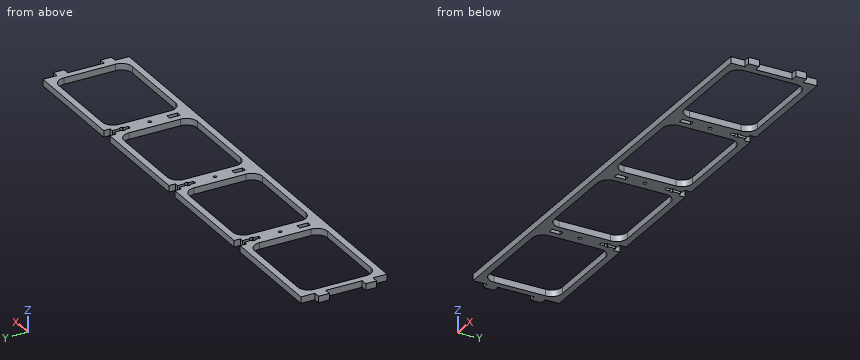
```python
from build123d import *

# Parameters (mm, degrees)
SKETCH1_W           = 428
SKETCH1_H           = 80
BOSS_EXTRUDE1_DEPTH = 6
CUT_EXTRUDE1_DEPTH  = 6
LPATTERN1_COUNT     = 4
LPATTERN1_PITCH     = 108.125
SKETCH3_R           = 1.6
SKETCH3_W           = 4.5
SKETCH3_H           = 10
CUT_EXTRUDE2_DEPTH  = 7
SKETCH4_W           = 6
SKETCH4_H           = 10
BOSS_EXTRUDE2_DEPTH = 6
SKETCH5_W           = 10
SKETCH5_H           = 6
CUT_EXTRUDE3_DEPTH  = 6
CUT_EXTRUDE4_REACH  = 8


with BuildPart() as part:
    # Sketch1 → Boss-Extrude1 (new body)
    with BuildSketch(Plane.XY):
        Rectangle(SKETCH1_W, SKETCH1_H)
    extrude(amount=BOSS_EXTRUDE1_DEPTH)

    # Sketch2 → Cut-Extrude1 (cut)
    with BuildSketch(Plane.XY.offset(6)):
        with BuildLine():
            Line((-116.375, -24), (-116.375, 24))
            ThreePointArc((-116.375, 24), (-119.303932188, 31.071067812), (-126.375, 34))
            Line((-126.375, 34), (-198, 34))
            ThreePointArc((-198, 34), (-205.071067812, 31.071067812), (-208, 24))
            Line((-208, 24), (-208, -24))
            ThreePointArc((-208, -24), (-205.071067812, -31.071067812), (-198, -34))
            Line((-198, -34), (-126.375, -34))
            ThreePointArc((-126.375, -34), (-119.303932188, -31.071067812), (-116.375, -24))
        make_face()
    cut_extrude1 = extrude(amount=-CUT_EXTRUDE1_DEPTH, mode=Mode.SUBTRACT)

    # LPattern1: Cut-Extrude1 ×4
    with Locations(*[(i * LPATTERN1_PITCH, 0, 0) for i in range(1, LPATTERN1_COUNT)]):
        add(cut_extrude1, mode=Mode.SUBTRACT)

    # Sketch3 → Cut-Extrude2 (cut, through all)
    with BuildSketch(Plane(origin=(0, 0, 0), x_dir=(-1, 0, 0), z_dir=(0, 0, -1))):
        with Locations((108.125, 0)):
            Circle(SKETCH3_R)
        Circle(SKETCH3_R)
        with Locations((-108.125, 0)):
            Circle(SKETCH3_R)
        with Locations((-108.125, -22)):
            Rectangle(SKETCH3_W, SKETCH3_H)
        with Locations((0, -22)):
            Rectangle(SKETCH3_W, SKETCH3_H)
        with Locations((108.125, -22)):
            Rectangle(SKETCH3_W, SKETCH3_H)
    extrude(amount=-CUT_EXTRUDE2_DEPTH, mode=Mode.SUBTRACT)

    # Sketch4 → Boss-Extrude2 (add)
    with BuildSketch(Plane(origin=(0, 0, 0), x_dir=(-1, 0, 0), z_dir=(0, 0, -1))):
        with Locations((-217, 22)):
            Rectangle(SKETCH4_W, SKETCH4_H)
        with Locations((-217, -22)):
            Rectangle(SKETCH4_W, SKETCH4_H)
        with Locations((217, -22)):
            Rectangle(SKETCH4_W, SKETCH4_H)
        with Locations((217, 22)):
            Rectangle(SKETCH4_W, SKETCH4_H)
    extrude(amount=-BOSS_EXTRUDE2_DEPTH)

    # Sketch5 → Cut-Extrude3 (cut)
    with BuildSketch(Plane(origin=(0, 40, 0), x_dir=(1, 0, 0), z_dir=(0, 1, 0))):
        with Locations((-108.125, -3)):
            Rectangle(SKETCH5_W, SKETCH5_H)
        with Locations((0, -3)):
            Rectangle(SKETCH5_W, SKETCH5_H)
        with Locations((108.125, -3)):
            Rectangle(SKETCH5_W, SKETCH5_H)
    extrude(amount=-CUT_EXTRUDE3_DEPTH, mode=Mode.SUBTRACT)

    # Sketch6 → Cut-Extrude4 (cut, up to next)
    with BuildSketch(Plane(origin=(0, 0, 0), x_dir=(-1, 0, 0), z_dir=(0, 0, -1)), mode=Mode.PRIVATE) as cut_extrude4_sk1:
        Polygon((-109.725, 34), (-109.725, 27), (-110.925, 27), (-110.925, 24), (-109.725, 24), (-109.725, 19), (-106.525, 19), (-106.525, 24), (-105.325, 24), (-105.325, 27), (-106.525, 27), (-106.525, 34), align=None)
    cut_extrude4_tool1 = extrude(cut_extrude4_sk1.sketch, amount=-CUT_EXTRUDE4_REACH, mode=Mode.PRIVATE) & part.part
    add(cut_extrude4_tool1.solids().sort_by_distance((108.125, 26.369565, 0))[0], mode=Mode.SUBTRACT)
    # Sketch6 → Cut-Extrude4 (cut, up to next)
    with BuildSketch(Plane(origin=(0, 0, 0), x_dir=(-1, 0, 0), z_dir=(0, 0, -1)), mode=Mode.PRIVATE) as cut_extrude4_sk2:
        Polygon((-1.595, 27), (-2.795, 27), (-2.795, 24), (-1.595, 24), (-1.595, 19), (1.605, 19), (1.605, 24), (2.805, 24), (2.805, 27), (1.605, 27), (1.605, 34), (-1.595, 34), align=None)
    cut_extrude4_tool2 = extrude(cut_extrude4_sk2.sketch, amount=-CUT_EXTRUDE4_REACH, mode=Mode.PRIVATE) & part.part
    add(cut_extrude4_tool2.solids().sort_by_distance((-0.005, 26.369565, 0))[0], mode=Mode.SUBTRACT)
    # Sketch6 → Cut-Extrude4 (cut, up to next)
    with BuildSketch(Plane(origin=(0, 0, 0), x_dir=(-1, 0, 0), z_dir=(0, 0, -1)), mode=Mode.PRIVATE) as cut_extrude4_sk3:
        Polygon((106.535, 34), (106.535, 27), (105.335, 27), (105.335, 24), (106.535, 24), (106.535, 19), (109.735, 19), (109.735, 24), (110.935, 24), (110.935, 27), (109.735, 27), (109.735, 34), align=None)
    cut_extrude4_tool3 = extrude(cut_extrude4_sk3.sketch, amount=-CUT_EXTRUDE4_REACH, mode=Mode.PRIVATE) & part.part
    add(cut_extrude4_tool3.solids().sort_by_distance((-108.135, 26.369565, 0))[0], mode=Mode.SUBTRACT)


solid = part.part
```
Geometry check sheet. Reference: the model listing, model coordinates, mm. Give positions to 0.01 mm unless a question says otherwise; leave off trailing zeros. Loops run counter-clockwise (first coordinate to the right, second up) from the corner with the lowest first, then second, coordinate; pieces in that order, holes last. Notation, with made-up numbers: M 36,4.25 L 66,4.25 A27 ccw 66,22.25 Z; hole C 28,86.25 d3. An arc over 180 degrees is marked long. Answer as CSV lines item,"result".
Item 1: Cross-section at B-B on z = 5.05. Count the separate pieces of the cut face and the enclosed holes in it, and give its area (3 significant figures).
Values:
separate pieces,"1"
enclosed holes,"10"
area,"9,400 mm²"
Item 2: Material ranges on line 1 (Y direction, x = 0, z = 1.8); line 2 (X direction, y = 14.5, z = 5) (3 decimals); line 3 (Y direction, x = -167, z = 0.85), recorded low to high.
Values:
line 1,"y = -40 to -27, -17 to -1.6, 1.6 to 19"
line 2,"x = -214 to -208, -116.375 to -99.875, -8.25 to 8.25, 99.875 to 116.375, 208 to 214"
line 3,"y = -40 to -34, 34 to 40"
Item 3: Cross-section at A-A on x = 178.5. Record the cut outline in (y, z).
Values:
outline,"M -40,0 L -34,0 L -34,6 L -40,6 Z; M 34,0 L 40,0 L 40,6 L 34,6 Z"
Item 4: Depth check by flat-ended pin: P1, Ø1, axis at x = 106, z = 2.5, coming from the +Y side; P2, Ø1.8, axis at y = 32, z = 4, coming from the -X side; P3, Ø3, axis at x = -218, z = 2, coming from the -Y side; P4, Ø2, axis at x = 107, y = -24.5, coming from the -Z side. Enter the tip coordinate at first touch or a pass-through.
Values:
P1,"stops at y = 34"
P2,"stops at x = -214"
P3,"stops at y = -27"
P4,"passes through"
